Could you check a few things on this model? Use its own coordinates, in mm. Face numbers are marked on the shaded views. A direction names the side the tool comes from. Give positions to 0.01 mm unless a question says otherwise; leave off trailing zeros. Loops run counter-clockwise (first coordinate to the right, second up) from the corner with the lowest first, then second, coordinate; pieces in that order, holes last. Notation, with made-up numbers: (85.25, 69) -> (135.25, 69) arc R32 ccw to (135.25, 98) -> close; hole circle Ø4 at (-18, 29). An arc over 180 degrees is marked (long way). Put each result on its own line as item: value.
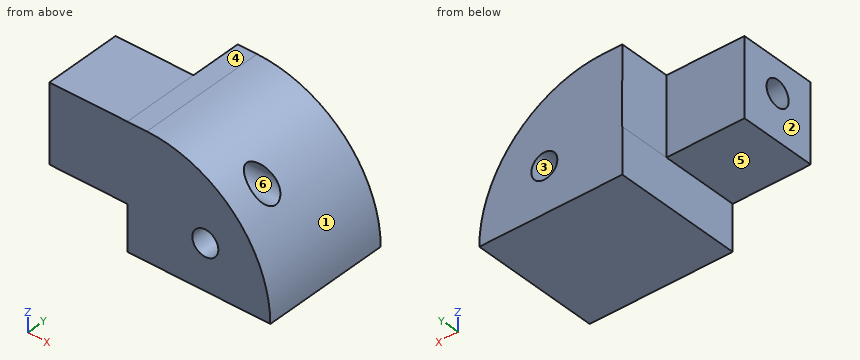
```python
from build123d import *

# Parameters (mm, degrees)
F1_DEPTH = 127
F3_DEPTH = 76.2
F4_W     = 76.2001280264
F4_H     = 50.8
F5_DEPTH = 76.2
F7_D     = 25.4
F9_D     = 25.4


with BuildPart() as f1:
    # F0 (on Front) → F1 (new body)
    with BuildSketch(Plane.XZ):
        Polygon((0, 0), (0, 120.65), (-19.05, 120.65), (-95.25, 120.5103173852), (-95.25, 0), (-19.05, 0), align=None)
        with BuildLine():
            ThreePointArc((120.65, 0), (85.3124331502, 85.3124331502), (0, 120.65))
            Line((0, 120.65), (0, 0))
            Line((0, 0), (120.65, 0))
        make_face()
    extrude(amount=F1_DEPTH)

    # F2 (on face) → F3 (cut)
    with BuildSketch(Plane(origin=(-95.25, 0, 0), x_dir=(0, -1, 0), z_dir=(-1, 0, 0))):
        Polygon((50.8, 44.45), (50.8, 120.5103173852), (0, 120.5103173852), (0, 0), (127, 0), (127, 44.45), align=None)
    extrude(amount=-F3_DEPTH, mode=Mode.SUBTRACT)

    # F4 (on face) → F5 (cut)
    with BuildSketch(Plane(origin=(-0.22122741, 0, 120.6845151206), x_dir=(0.9999983199, 0, 0.0018331021), z_dir=(-0.0018331021, 0, 0.9999983199))):
        with Locations((-56.9288682381, -25.4)):
            Rectangle(F4_W, F4_H)
    extrude(amount=-F5_DEPTH, mode=Mode.SUBTRACT)

    # F7 (through all)
    with Locations(Plane(origin=(-95.25, 0, 0), x_dir=(0, -1, 0), z_dir=(-1, 0, 0))):
        with Locations((88.9, 88.7603173852)):
            Hole(F7_D / 2)

    # F9 (through all)
    with Locations(Plane.XZ.offset(127)):
        with Locations((57.15, 44.45)):
            Hole(F9_D / 2)


solid = f1.part
```
1. I'm going to push flat-ended pins straight in: pin 1 (4 mm diameter, centred on x = 65, y = -68.5, fed in from +Z); pin 2 (15 mm diameter, centred on x = 57.15, z = 44.45, fed in from -Y); pin 3 (23 mm diameter, centred on x = -67.5, y = -78.5, fed in from -Z); pin 4 (4 mm diameter, centred on x = -50.5, z = 69.5, fed in from +Y). Where does each tip first touch, or does it pass through?
Recorded:
pin 1: stops at z = 102.9
pin 2: passes through
pin 3: stops at z = 44.45
pin 4: stops at y = -50.8
2. If we section it at C-C (y = -88.9): List the corners of the cut face in (x, z) for me.
Recorded:
outline: (-95.25, 44.45) -> (-19.05, 44.45) -> (-19.05, 0) -> (120.65, 0) arc R120.65 ccw to (93.65, 76.06) -> (-95.25, 76.06) -> close; (-95.25, 101.46) -> (65.29, 101.46) arc R120.65 ccw to (0, 120.65) -> (-19.05, 120.65) -> (-95.25, 120.51) -> close; hole circle Ø25.4 at (57.15, 44.45)
3. If we section it at B-B (y = -116.5): List the corners of the cut face in (x, z) for me, then the cut area to 3 significant figures.
Recorded:
outline: (-95.25, 44.45) -> (-19.05, 44.45) -> (-19.05, 0) -> (120.65, 0) arc R120.65 ccw to (0, 120.65) -> (-19.05, 120.65) -> (-95.25, 120.51) -> close; hole circle Ø25.4 at (57.15, 44.45)
area: 19,000 mm^2
4. For the marked faces 5 and 6, which set-ups out of +Z, -Z, +X, -X, +Y, -Y let a thin tool reach every point of the face, with its end or its side?
Recorded:
face 5: -Z, -X, +Y, -Y
face 6: +X, -X
5. Thinking about a two-plate mould opening in X: for the marked faces 1, 2, 3 and 4, which applies, pulls with the +X half, pulls with the -X half, needs draft (parallel to the pull), parting line crosses it, or undercut?
Recorded:
face 1: pulls with the +X half
face 2: pulls with the -X half
face 3: undercut
face 4: needs draft
6. If we section it at D-D (z = 83): List the corners of the cut face in (x, y) for me.
Recorded:
outline: (-95.25, -127) -> (87.56, -127) -> (87.56, -100.22) -> (-95.25, -100.22) -> close; (-95.25, -77.58) -> (87.56, -77.58) -> (87.56, 0) -> (-18.98, 0) -> (-18.98, -50.8) -> (-95.25, -50.8) -> close
7. I need wall thicknesses on line 1 (Z direction, x = -14, y = -88); line 2 (Z direction, x = 57, y = -59); line 3 (Z direction, x = 1, y = -10). Which ranges of each line are inside material? Lowest first, please.
Recorded:
line 1: z = 0 to 76.09, 101.43 to 120.65
line 2: z = 0 to 31.75, 57.15 to 106.34
line 3: z = 0 to 120.65
8. If we section it at A-A (x = 47): List the corners of the cut face in (y, z) for me, then the cut area to 3 significant figures.
Recorded:
outline: (-127, 0) -> (0, 0) -> (0, 36.82) -> (-127, 36.82) -> close; (-127, 52.08) -> (0, 52.08) -> (0, 111.12) -> (-127, 111.12) -> close; hole circle Ø25.4 at (-88.9, 88.76)
area: 11,700 mm^2
